```python
from build123d import *

# Parameters (mm, degrees)
ESBO_O1_R                = 3
ESBO_O1_R_2              = 1.625
ESBO_O1_W                = 30
ESBO_O1_H                = 3
RESSALTO_EXTRUS_O1_DEPTH = 3
FILETE1_R                = 5


with BuildPart() as part:
    # Esboço1 → Ressalto-extrusão1 (new body)
    with BuildSketch(Plane.XY):
        Polygon((160, -20), (215, -20), (215, -70.5), (250, -70.5), (250, -20), (250, 22.5), (229.5, 22.5), (199.5, 22.5), (179, 22.5), (179, 0), (0, 0), (0, -20), (50, -20), (50, -17), (80, -17), (80, -20), (130, -20), (130, -17), (160, -17), align=None)
        with Locations((232.5, -60.5)):
            Circle(ESBO_O1_R, mode=Mode.SUBTRACT)
        with Locations((232.5, -44.5)):
            Circle(ESBO_O1_R, mode=Mode.SUBTRACT)
        with BuildLine():
            ThreePointArc((124, -9.5), (122.5, -8), (124, -6.5))
            Line((124, -6.5), (159, -6.5))
            ThreePointArc((159, -6.5), (160.5, -8), (159, -9.5))
            Line((159, -9.5), (124, -9.5))
        make_face(mode=Mode.SUBTRACT)
        with Locations((189.75, -5)):
            Circle(ESBO_O1_R_2, mode=Mode.SUBTRACT)
        Polygon((194, 1.5), (194, 10.5), (235, 10.5), (235, 1.5), (240, 1.5), (240, -1.5), (235, -1.5), (235, -10.5), (194, -10.5), (194, -1.5), (189, -1.5), (189, 1.5), align=None, mode=Mode.SUBTRACT)
        with Locations((239.25, -5)):
            Circle(ESBO_O1_R_2, mode=Mode.SUBTRACT)
        with Locations((189.75, 5)):
            Circle(ESBO_O1_R_2, mode=Mode.SUBTRACT)
        with Locations((239.25, 5)):
            Circle(ESBO_O1_R_2, mode=Mode.SUBTRACT)
        with Locations((214.5, 24)):
            Rectangle(ESBO_O1_W, ESBO_O1_H)
    extrude(amount=RESSALTO_EXTRUS_O1_DEPTH)

    # Filete1
    filete1_edges = [part.edges().sort_by_distance(p)[0] for p in [
        (250, 22.5, 1.5),
        (250, -70.5, 1.5),
        (215, -70.5, 1.5),
        (215, -20, 1.5),
        (0, 0, 1.5),
        (179, 0, 1.5),
        (179, 22.5, 1.5),
    ]]
    fillet(filete1_edges, radius=FILETE1_R)


solid = part.part
```
The model under review builds one solid part; all positions refer to its coordinate system, in mm. Coordinates: 2 decimals unless noted, no trailing zeros. Write each loop counter-clockwise with the first axis right and the second up, starting at its lowest first coordinate (ties: lowest second). Pieces come first, ordered by that corner, then holes.
1) We need section D-D on z = 2. Count the separate pieces of the cut face and the enclosed holes in it, then the cut area to 3 significant figures.
2) We need section A-A on x = 232.5. State the section outline as (y, z) points.
3) We need section C-C on x = 141. State the section outline as (y, z) points.
4) To check wall thickness, follow probe 1 along Y at (x, z) = (239.25, 1) (3 decimals); probe 2 along Y at (x, z) = (232.5, 1.9); probe 3 along Y at (x, z) = (198, 1.45). State the ranges of each line that lie inside material, in increasing order.
5) We need section B-B on y = -44.5. State the section outline as (x, z) points, then the cut area to 3 significant figures.
6) The part is to be moulded in two halves that separate along Y. For faces 1 (the face through (213, -21, 2)), 2 (the face through (229.5, -44.4, 1.5)), 3 (the face through (161, -15, 0)), say which applies: pulls with the +Y half, pulls with the -Y half, needs draft (parallel to the pull), parting line crosses it, or undercut.
7) Clearance check with flat-ended pins moving along their axes: pin 1 Ø1.9 at (x, y) = (239.25, 5) entering from -Z; pin 2 Ø1.5 at (x, z) = (210.5, 1.5) entering from -Y; pin 3 Ø12 at (x, y) = (207.5, 6.5) entering from -Z; pin 4 Ø1.5 at (y, z) = (23.5, 1.5) entering from -X. State where each tip first meets the part, or that it passes through.
Answer list:
1. separate pieces: 1
1. enclosed holes: 8
1. area: 7,170 mm2
2. outline: (-70.5, 0) - (-63.5, 0) - (-63.5, 3) - (-70.5, 3) - close; (-57.5, 0) - (-47.5, 0) - (-47.5, 3) - (-57.5, 3) - close; (-41.5, 0) - (-10.5, 0) - (-10.5, 3) - (-41.5, 3) - close; (10.5, 0) - (22.5, 0) - (22.5, 3) - (10.5, 3) - close
3. outline: (-17, 0) - (-9.5, 0) - (-9.5, 3) - (-17, 3) - close; (-6.5, 0) - (0, 0) - (0, 3) - (-6.5, 3) - close
4. probe 1: y = -70.5 to -6.625, -3.375 to -1.5, 1.5 to 3.375, 6.625 to 22.5
4. probe 2: y = -70.5 to -63.5, -57.5 to -47.5, -41.5 to -10.5, 10.5 to 22.5
4. probe 3: y = -20 to -10.5, 10.5 to 22.5
5. outline: (215, 0) - (229.5, 0) - (229.5, 3) - (215, 3) - close; (235.5, 0) - (250, 0) - (250, 3) - (235.5, 3) - close
5. area: 87.0 mm2
6. face 1: pulls with the -Y half
6. face 2: undercut
6. face 3: needs draft
7. pin 1: passes through
7. pin 2: stops at y = -20.16
7. pin 3: stops at z = 0
7. pin 4: stops at x = 199.5
